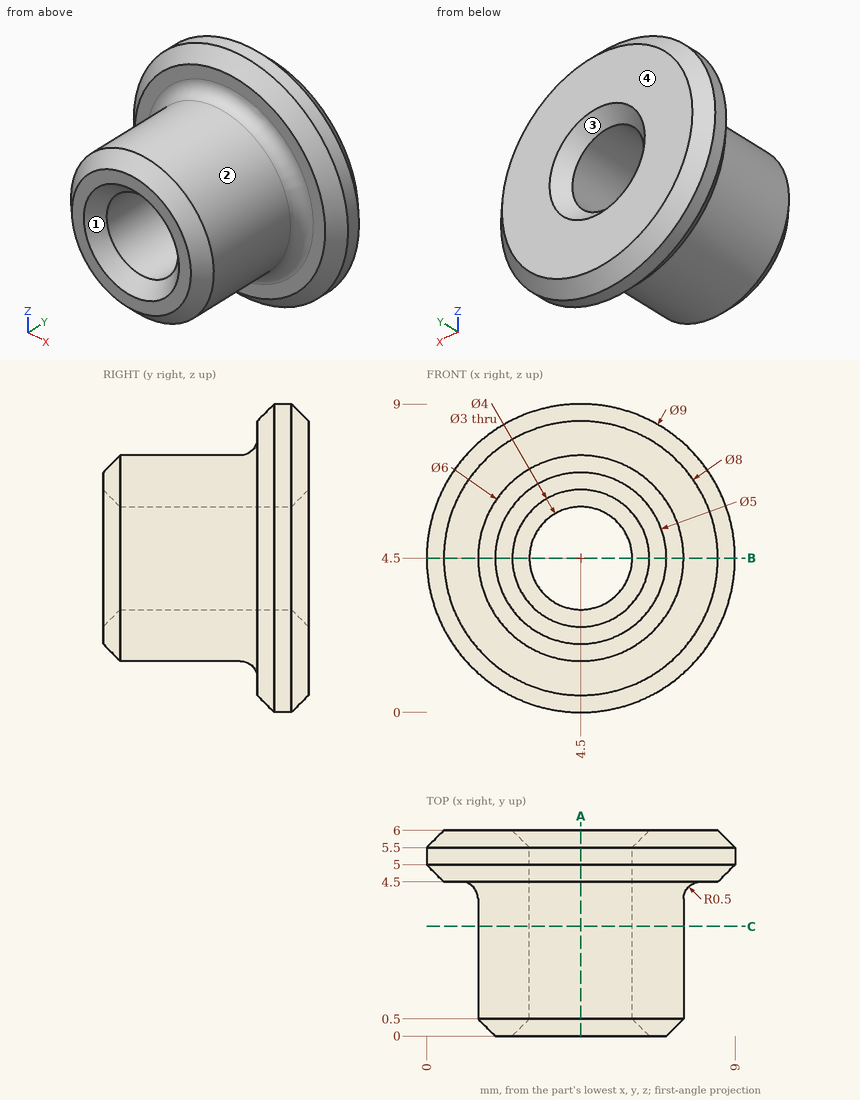
Could you check a few things on this drawing? It's one solid part, dimensions in mm from its lowest x, y, z. Round coordinates to 2 decimals unless told otherwise and drop trailing zeros. Order: outer loops, then holes, each group sorted by start corner. A loop starts at its lowest first (then second) coordinate and runs counter-clockwise, first axis right, second up. Notation, with made-up numbers: M -6.75,77.5 L 48.25,77.5 A26 ccw 48.25,98.5 Z; hole C 83,16 d7. An arc over 180 degrees is marked long. One line per question, with ' | ' between items.
1) Imagine slicing it at C-C, the plane y = 3.2. Write out the boundary of the cut face in (x, z), plus the area to 3 significant figures.
Checked values:
outline: C 4.5,4.5 d6; hole C 4.5,4.5 d3 | area: 21.2 mm²
2) I'm going to push flat-ended pins straight in: pin 1 Ø2 at (x, z) = (4, 4) entering from +Y; pin 2 Ø1 at (y, z) = (1, 6.5) entering from +X; pin 3 Ø1 at (x, y) = (1.5, 1.5) entering from +Z. Where does each tip first touch, or does it pass through?
Checked values:
pin 1: stops at y = 5.71 | pin 2: stops at x = 7.1 | pin 3: stops at z = 6.16
3) We'd pull the mould along Z, two halves only. Please class the marked faces 1, 2, 3 and 4: released by +Z, released by -Z, zero draft, split by the parting line, or undercut.
Checked values:
face 1: undercut | face 2: split by the parting line | face 3: undercut | face 4: zero draft
4) Imagine slicing it at B-B, the plane z = 4.5. Write out the boundary of the cut face in (x, y).
Checked values:
outline: M 0,5 L 0.5,4.5 L 1,4.5 A0.5 cw 1.5,4 L 1.5,0.5 L 2,0 L 2.5,0 L 3,0.5 L 3,5.5 L 2.5,6 L 0.5,6 L 0,5.5 Z; M 6,0.5 L 6.5,0 L 7,0 L 7.5,0.5 L 7.5,4 A0.5 cw 8,4.5 L 8.5,4.5 L 9,5 L 9,5.5 L 8.5,6 L 6.5,6 L 6,5.5 Z
5) Imagine slicing it at A-A, the plane x = 4.5. Write out the boundary of the cut face in (y, z).
Checked values:
outline: M 0,2 L 0.5,1.5 L 4,1.5 A0.5 cw 4.5,1 L 4.5,0.5 L 5,0 L 5.5,0 L 6,0.5 L 6,2.5 L 5.5,3 L 0.5,3 L 0,2.5 Z; M 0,6.5 L 0.5,6 L 5.5,6 L 6,6.5 L 6,8.5 L 5.5,9 L 5,9 L 4.5,8.5 L 4.5,8 A0.5 cw 4,7.5 L 0.5,7.5 L 0,7 Z
6) I need wall thicknesses on line 1 (Z direction, x = 4.5, y = 3.05); line 2 (Y direction, x = 5.5, z = 1). Which ranges of each line are inside material? Lowest first, please.
Checked values:
line 1: z = 1.5 to 3, 6 to 7.5 | line 2: y = 4.5 to 6
